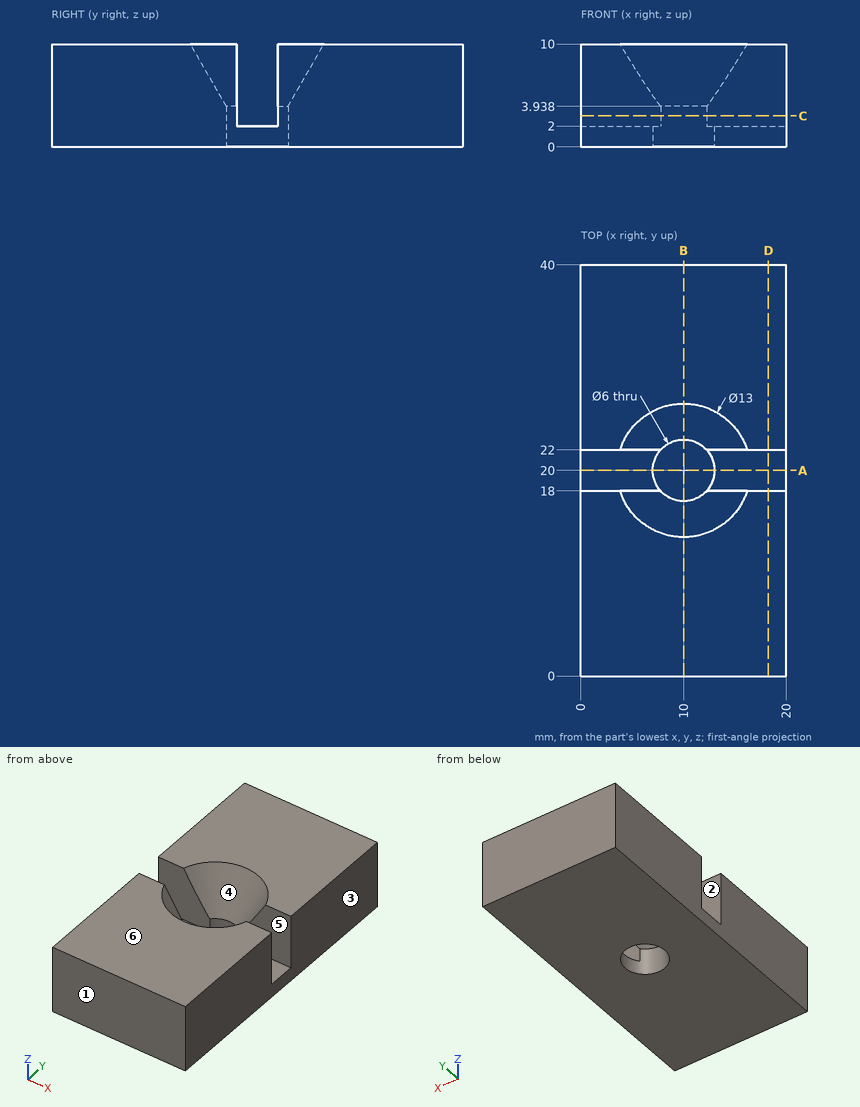
Design review of the part shown in the three views and the two pictorial views. Dimensions are in mm from the part's minimum x, y and z. A direction names the side the tool comes from. Round coordinates to 2 decimals unless told otherwise and drop trailing zeros. Loops run counter-clockwise (first coordinate to the right, second up) from the corner with the lowest first, then second, coordinate; pieces in that order, holes last.
1) Clearance check with flat-ended pins moving along their axes: P1, Ø4, axis at x = 11, y = 20.5, coming from the +Z side; P2, Ø5.5, axis at x = 10, y = 20, coming from the -Z side; P3, Ø2, axis at x = 17.5, y = 20, coming from the +Z side. State where each tip first meets the part, or that it passes through.
Values follow:
P1: stops at z = 4.05
P2: passes through
P3: stops at z = 2
2) Consider section A-A on y = 20. State the section outline as (x, z) points.
Values follow:
outline: (0, 0) - (7, 0) - (7, 2) - (0, 2) - close; (13, 0) - (20, 0) - (20, 2) - (13, 2) - close
3) Tool access review of the marked faces 4, 5 and 6: name each direction out of +Z, -Z, +X, -X, +Y, -Y from which nothing blocks a thin tool from reaching the whole face with its end or side.
Values follow:
face 4: +Z
face 5: +Z, +X, -X
face 6: +Z, +X, -X, +Y, -Y
4) Wall thickness on line 1 along Y through (x, z) = (3.5, 4); line 2 along Y through (x, z) = (10, 2.95); line 3 along X through (y, z) = (20, 1.9): over which ranges is each line inside the solid? List them lowest first.
Values follow:
line 1: y = 0 to 18, 22 to 40
line 2: y = 0 to 17, 23 to 40
line 3: x = 0 to 7, 13 to 20
5) Consider section C-C on z = 3. State the section outline as (x, y) points, then the cut area to 3 significant figures.
Values follow:
outline: (0, 0) - (20, 0) - (20, 18) - (12.24, 18) arc R3 cw to (7.76, 18) - (0, 18) - close; (0, 22) - (7.76, 22) arc R3 cw to (12.24, 22) - (20, 22) - (20, 40) - (0, 40) - close
area: 714 mm2
6) Consider section B-B on x = 10. State the section outline as (y, z) points, then the cut area to 3 significant figures.
Values follow:
outline: (0, 0) - (17, 0) - (17, 3.94) - (13.5, 10) - (0, 10) - close; (23, 0) - (40, 0) - (40, 10) - (26.5, 10) - (23, 3.94) - close
area: 319 mm2
7) The part is to be moulded in two halves that separate along Y. For the marked faces 1, 2 and 3, say which applies: pulls with the +Y half, pulls with the -Y half, needs draft (parallel to the pull), parting line crosses it, or undercut.
Values follow:
face 1: pulls with the -Y half
face 2: undercut
face 3: needs draft
8) Consider section D-D on x = 18.25. State the section outline as (y, z) points, then the cut area to 3 significant figures.
Values follow:
outline: (0, 0) - (40, 0) - (40, 10) - (22, 10) - (22, 2) - (18, 2) - (18, 10) - (0, 10) - close
area: 368 mm2
